Autodesk Inventor part; units mm, degrees
ref_plane "YZ Plane" through (0, 0, 0) normal (1, 0, 0) x (0, 1, 0)
ref_plane "XZ Plane" through (0, 0, 0) normal (0, 1, 0) x (-1, 0, 0)
ref_plane "XY Plane" through (0, 0, 0) normal (0, 0, 1) x (1, 0, 0)
sketch "Sketch1" plane through (0, 0, 0) normal (0, 1, 0) x (-1, 0, 0)
  line L0 (0, 0) -> (0, 14)
  line L1 (10.1716, 14) -> (16.458, -5.3475)
  line L2 (16.458, -5.3475) -> (0, -17.305)
  line L3 (0, -17.305) -> (-16.458, -5.3475)
  line L4 (-16.458, -5.3475) -> (-10.1716, 14)
  line L5 (-10.1716, 14) -> (10.1716, 14)
  line L6 (0, -17.305) -> (10.1716, 14)
  line L7 (-10.1716, 14) -> (0, -17.305)
  line L8 (16.458, -5.3475) -> (-16.458, -5.3475)
  line L9 (-16.458, -5.3475) -> (10.1716, 14)
  line L10 (16.458, -5.3475) -> (-10.1716, 14)
  line L11 (0, 0) -> (0, -4.5)
  line L12 (-3.2694, -4.5) -> (-5.2901, 1.7188)
  line L13 (-5.2901, 1.7188) -> (0, 5.5623)
  line L14 (0, 5.5623) -> (5.2901, 1.7188)
  line L15 (5.2901, 1.7188) -> (3.2694, -4.5)
  line L16 (3.2694, -4.5) -> (-3.2694, -4.5)
  point P0 (-3.8852, -5.3475)
  point P1 (3.8852, -5.3475)
  point P2 (6.2864, 2.0426)
  point P3 (0, 6.6099)
  point P4 (-6.2864, 2.0426)
  dimension "d0" = 14
  dimension "d3" = 4.5
extrude "Extrusion2" add sketch "Sketch1" along normal blind 32 contours L10 L6 L8 L7 L9 | L9 L7 L10 | L9 L6 L10 | L7 L8 L9 | L10 L8 L6 | L8 L6 L7
properties part number "Star"
Here's how the part is built. I have some questions about the finished solid (model axes, mm). A direction names the side the tool comes from. Give positions to 0.01 mm unless a question says otherwise; leave off trailing zeros. Loops run counter-clockwise (first coordinate to the right, second up) from the corner with the lowest first, then second, coordinate; pieces in that order, holes last. Notation, with made-up numbers: (-16.5, -5) -> (22.5, -5) arc R22 ccw to (22.5, 11) -> close; hole circle Ø2 at (-15.5, 70). An arc over 180 degrees is marked (long way). Use one line per item in the form item = value. Start each with the question number.
1) Which directions (+Z, -Z, +X, -X, +Y, -Y) give clear straight access to the entire face, cutting with the end or side of a thin tool? Please do faces 1 (the face through (-8.202, 15.776, 7.938)), 2 (the face through (10, 16, -5.348)), 3 (the face through (-10, 16, -5.348)), 4 (the face through (8.256, 15.776, 8.105)), 5 (the face through (5.01, 15.78, 10.25)).
2) Imagine slicing it at B-B (y = 29). Please give me the cut outline in (x, z) (1 decimal).
3) Imagine slicing it at A-A (z = -0.5). Please give me the cut outline in (x, y), then the cut area to 3 significant figures.
4) Imagine slicing it at C-C (x = 8). Please give me the cut outline in (y, z).
5) Imagine slicing it at D-D (x = -13). Please give me the cut outline in (y, z).
6) For P1, Ø5, axis at x = -0.5, y = 18.5, coming from the +Z side; P2, Ø5, axis at y = 21.5, z = 10.5, coming from the -X side; P3, Ø1, axis at y = 14, z = 4, coming from the +X side, each with a flat end and sliding along its axis, tell me the tip position at first contact or that it passes through.
7) Please list where these lines run through material, in increasing order: line 1 along X through (y, z) = (21, 9); line 2 along X through (y, z) = (16, 1); line 3 along Z through (x, y) = (-6, 27).
8) Thinking about a two-plate mould opening in X: for faces 6 (the face through (4.266, 15.776, -1.434)), 7 (the face through (11.44, 15.78, -1.7)), 8 (the face through (-11.44, 15.78, -1.7)), which applies, +X half, -X half, draft (parallel to the pull), parting line (faces both ways), or undercut?
Check values:
q1.face_1 = -X, +Y, -Y
q1.face_2 = -Z, +X, +Y, -Y
q1.face_3 = -Z, -X, +Y, -Y
q1.face_4 = +X, +Y, -Y
q1.face_5 = +Z, +Y, -Y
q2.outline = (-16.5, -5.3) -> (-3.9, -5.3) -> (0, -17.3) -> (3.9, -5.3) -> (16.5, -5.3) -> (6.3, 2) -> (10.2, 14) -> (0, 6.6) -> (-10.2, 14) -> (-6.3, 2) -> close; hole (-5.3, 1.7) -> (-3.3, -4.5) -> (3.3, -4.5) -> (5.3, 1.7) -> (0, 5.6) -> close
q3.outline = (-9.79, 0) -> (-4.57, 0) -> (-4.57, 32) -> (-9.79, 32) -> close; (4.57, 0) -> (9.79, 0) -> (9.79, 32) -> (4.57, 32) -> close
q3.area = 334 mm^2
q4.outline = (0, -5.35) -> (32, -5.35) -> (32, 0.8) -> (0, 0.8) -> close; (0, 7.32) -> (32, 7.32) -> (32, 12.42) -> (0, 12.42) -> close
q5.outline = (0, -5.35) -> (32, -5.35) -> (32, -2.84) -> (0, -2.84) -> close
q6.P1 = 8.79
q6.P2 = -9.85
q6.P3 = 7.08
q7.line_1 = -8.55 to -3.29, 3.29 to 8.55
q7.line_2 = -7.72 to -5.06, 5.06 to 7.72
q7.line_3 = -5.35 to 10.97
q8.face_6 = undercut
q8.face_7 = +X half
q8.face_8 = -X half
